Read the model definition and answer for the solid it produces. Units are mm, in the model's axes. Round coordinates to 2 decimals unless told otherwise and drop trailing zeros. Loops run counter-clockwise (first coordinate to the right, second up) from the corner with the lowest first, then second, coordinate; pieces in that order, holes last. Notation, with made-up numbers: M -22,62.25 L -2,62.25 A32 ccw -2,98.25 Z; hole C 59,65 d8. An arc over 180 degrees is marked long. Write each question's results on one line, items separated by ' | '.
from build123d import *

# Parameters (mm, degrees)
F0_W     = 152.4
F0_H     = 152.4
F0_R     = 3.96875
F1_DEPTH = 6.35


with BuildPart() as f1:
    # F0 (on Top) → F1 (new body)
    with BuildSketch(Plane.XY):
        with Locations((76.2, 76.2)):
            Rectangle(F0_W, F0_H)
        with Locations((7.9375, 8.49987)):
            Circle(F0_R, mode=Mode.SUBTRACT)
        with BuildLine():
            Line((133.35, 12.7), (19.05, 12.7))
            ThreePointArc((19.05, 12.7), (14.559872, 14.559872), (12.7, 19.05))
            Line((12.7, 19.05), (12.7, 133.35))
            ThreePointArc((12.7, 133.35), (14.559872, 137.840128), (19.05, 139.7))
            Line((19.05, 139.7), (133.35, 139.7))
            ThreePointArc((133.35, 139.7), (137.840128, 137.840128), (139.7, 133.35))
            Line((139.7, 133.35), (139.7, 19.05))
            ThreePointArc((139.7, 19.05), (137.840128, 14.559872), (133.35, 12.7))
        make_face(mode=Mode.SUBTRACT)
        with Locations((144.4625, 8.49987)):
            Circle(F0_R, mode=Mode.SUBTRACT)
        with Locations((7.9375, 145.02487)):
            Circle(F0_R, mode=Mode.SUBTRACT)
        with Locations((144.4625, 145.02487)):
            Circle(F0_R, mode=Mode.SUBTRACT)
    extrude(amount=F1_DEPTH)


solid = f1.part
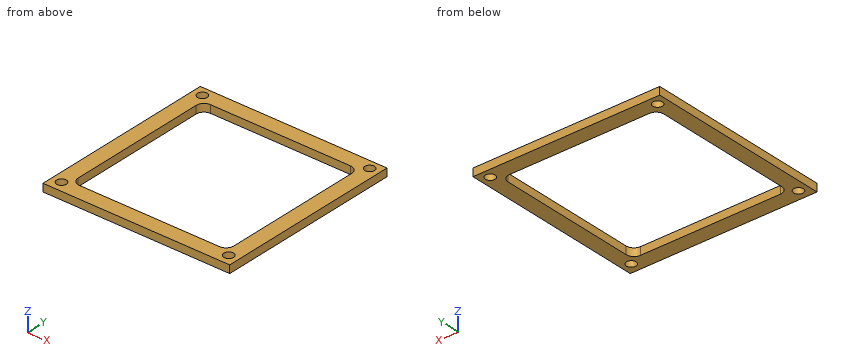
Item 1: The part is cut by section A-A (x = 42). Determine the outline of the cut face in (y, z), plus the area to 3 significant figures.
Outcome:
outline: M 0,0 L 12.7,0 L 12.7,6.35 L 0,6.35 Z; M 139.7,0 L 152.4,0 L 152.4,6.35 L 139.7,6.35 Z | area: 161 mm2
Item 2: The part is cut by section C-C (z = 2.25). Determine the outline of the cut face in (x, y), plus the area to 3 significant figures.
Outcome:
outline: M 0,0 L 152.4,0 L 152.4,152.4 L 0,152.4 Z; hole C 7.94,8.5 d7.94; hole C 7.94,145.02 d7.94; hole M 12.7,19.05 A6.35 ccw 19.05,12.7 L 133.35,12.7 A6.35 ccw 139.7,19.05 L 139.7,133.35 A6.35 ccw 133.35,139.7 L 19.05,139.7 A6.35 ccw 12.7,133.35 Z; hole C 144.46,8.5 d7.94; hole C 144.46,145.02 d7.94 | area: 6,930 mm2
Item 3: Straight lines are drawn through the part: line 1 (Y direction, x = 131.5, z = 5); line 2 (Y direction, x = 141, z = 0.75). For each, find the intervals that lie inside material, in ascending order.
Outcome:
line 1: y = 0 to 12.7, 139.7 to 152.4 | line 2: y = 0 to 6.56, 10.44 to 143.09, 146.96 to 152.4
